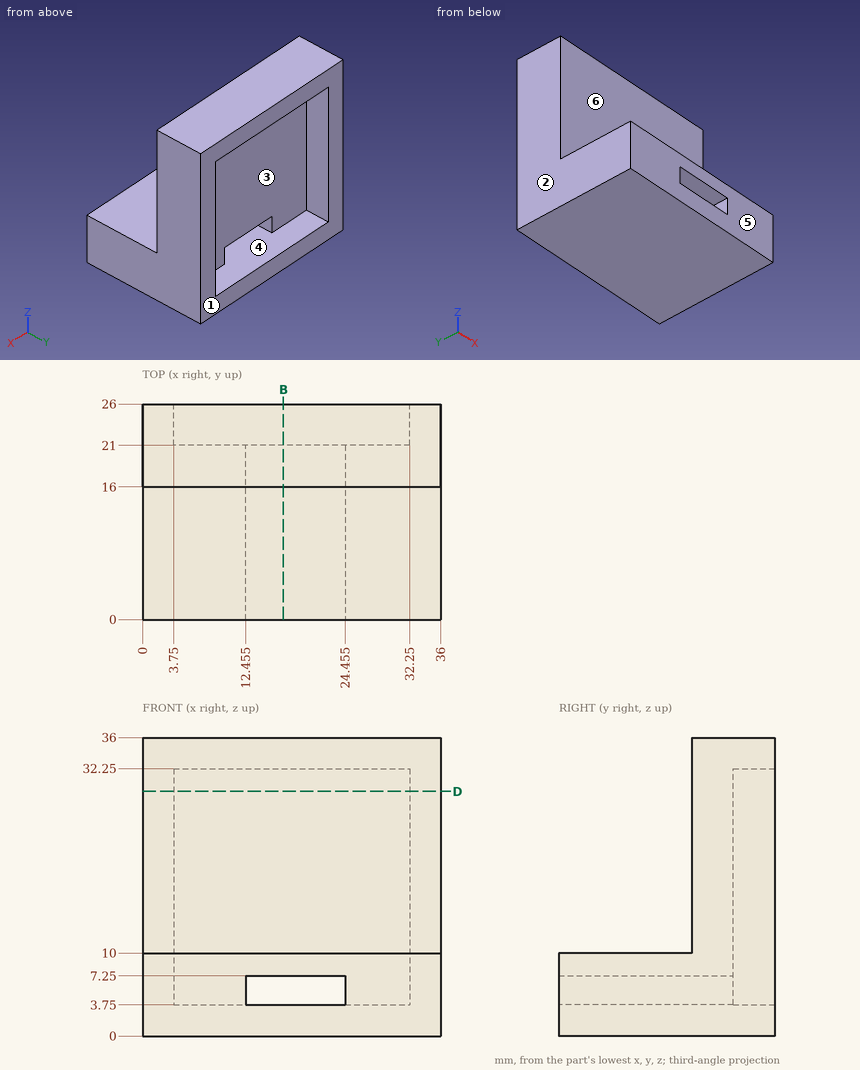
Answer from the drawing. Dimensions are ordinates in mm from the lowest x, y and z of the part. A direction names the side the tool comes from. Coordinates: 2 decimals unless noted, no trailing zeros. Write each loop counter-clockwise with the first axis right and the second up, starting at its lowest first coordinate (ties: lowest second). Pieces come first, ordered by that corner, then holes. Notation, with made-up numbers: M 68,59 L 76,59 A8 ccw 76,71 Z; hole C -35,73 d10. An arc over 180 degrees is marked long. Put each result on its own line as item: value. Start each with the question number.
1. Flat-ended cylindrical pins translate along their axes: P1, Ø5, axis at y = 14, z = 32, coming from the +X side; P2, Ø4, axis at x = 6.5, z = 18, coming from the +Y side; P3, Ø8, axis at x = 22.5, y = 4.5, coming from the +Z side; P4, Ø12, axis at y = 8.5, z = 26, coming from the -X side. Find the tip coordinate at first contact, or state that the pin passes through.
2. A cutting plane is placed at D-D on z = 29.5. Write down the section's boundary in (x, y).
3. Which of the six approach directions +Z, -Z, +X, -X, +Y, -Y give full straight-line access (tool end or side, diameter ignored) to the marked faces 4, 5 and 6?
4. For a pull along X with two mould halves and no side action, classify the marked faces 1, 2 and 3 as pulls with the +X half, pulls with the -X half, needs draft (parallel to the pull), parting line crosses it, or undercut.
5. A cutting plane is placed at B-B on x = 17. Write down the section's boundary in (y, z), then the cut area to 3 significant figures.
6. Consider line 1 (X direction, y = 23.25, z = 10); line 2 (Z direction, x = 12.5, y = 4.5); line 3 (Z direction, x = 21, y = 16.5). Determine where each line is inside the solid, lowest interval first. Write a range as from..to.
Resolved:
1. P1: stops at x = 36
1. P2: stops at y = 21
1. P3: stops at z = 10
1. P4: passes through
2. outline: M 0,16 L 36,16 L 36,26 L 32.25,26 L 32.25,21 L 3.75,21 L 3.75,26 L 0,26 Z
3. face 4: +Y
3. face 5: +Z, -Z, +X, -X, -Y
3. face 6: +Z, +X, -X, -Y
4. face 1: needs draft
4. face 2: pulls with the -X half
4. face 3: undercut
5. outline: M 0,0 L 26,0 L 26,3.75 L 0,3.75 Z; M 0,7.25 L 21,7.25 L 21,32.25 L 26,32.25 L 26,36 L 16,36 L 16,10 L 0,10 Z
5. area: 304 mm2
6. line 1: x = 0..3.75, 32.25..36
6. line 2: z = 0..3.75, 7.25..10
6. line 3: z = 0..3.75, 7.25..36
